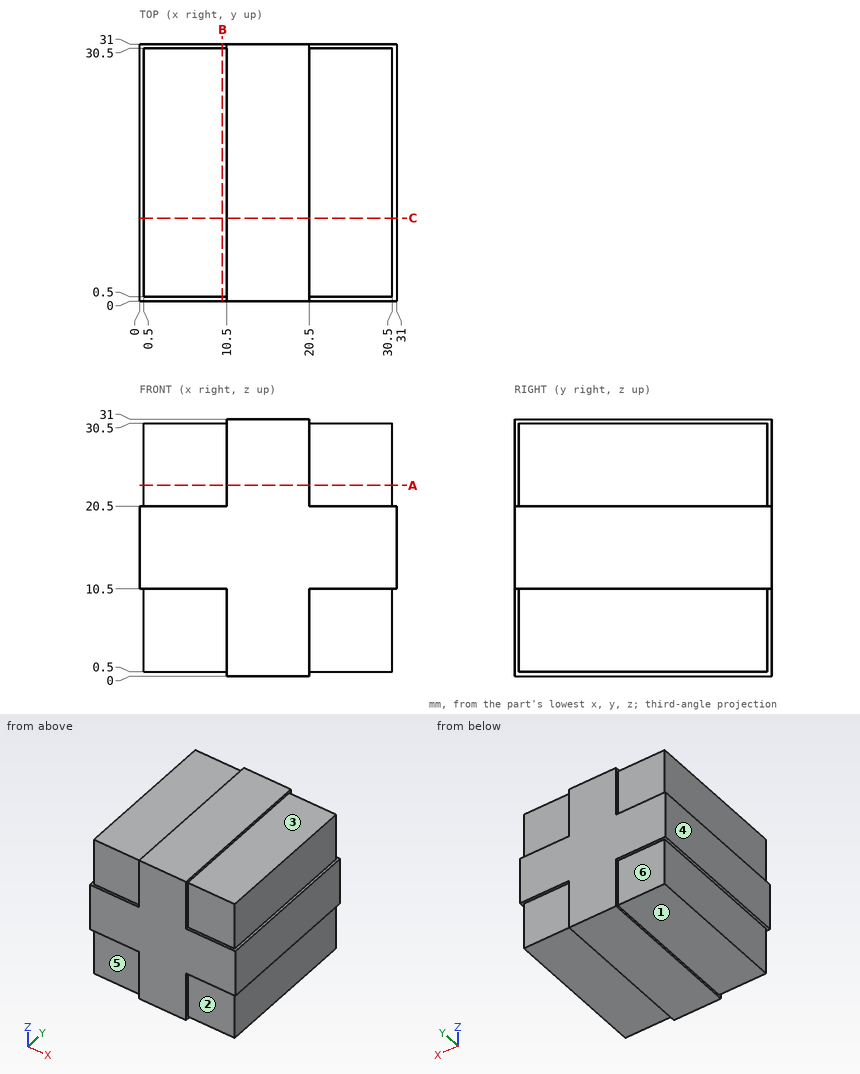
Geometry check sheet. Reference: drawing and pictorial views, mm from the part's lowest x, y, z. A direction names the side the tool comes from. Coordinates: 2 decimals unless noted, no trailing zeros. Order: outer loops, then holes, each group sorted by start corner. A loop starts at its lowest first (then second) coordinate and runs counter-clockwise, first axis right, second up. Notation, with made-up numbers: (11.25, 30) -> (55.25, 30) arc R18 ccw to (55.25, 37) -> close; hole circle Ø10 at (21.25, 79.5). An arc over 180 degrees is marked (long way). Put each result on its own line as item: value. Start each with the question number.
1) Cross-section at C-C (y = 10). Enter the section's corners in (x, z), plus the area to 3 significant figures.
2) Cross-section at B-B (x = 10). Enter the section's corners in (y, z), plus the area to 3 significant figures.
3) Cross-section at A-A (z = 23). Enter the section's corners in (x, y).
4) Release check for a two-part mould opening along Y. For the marked faces 4, 5 and 6 record: pulls with the +Y half, pulls with the -Y half, needs draft (parallel to the pull), parting line crosses it, or undercut.
5) Material ranges on L1, parallel to Y at x = 30, z = 8.5, recorded low to high.
6) Tool access check on the marked faces 1, 2 and 3. Record the directions out of +Z, -Z, +X, -X, +Y, -Y that give a thin tool (end or side, any length) a straight path to the whole face; none if there is none.
7) Go/stop test with flat-tipped pins: pin 1 (3 mm diameter, centred on x = 6.5, z = 6.5, fed in from +Y); pin 2 (12 mm diameter, centred on x = 15.5, z = 22, fed in from -Y); pin 3 (11 mm diameter, centred on x = 27, z = 3.5, fed in from -Y); pin 4 (3 mm diameter, centred on y = 8.5, z = 7.5, fed in from -X). Record where each tip stops, or that it passes through.
Geometry check:
1. outline: (0, 10.5) -> (0.5, 10.5) -> (0.5, 0.5) -> (10.5, 0.5) -> (10.5, 0) -> (20.5, 0) -> (20.5, 0.5) -> (30.5, 0.5) -> (30.5, 10.5) -> (31, 10.5) -> (31, 20.5) -> (30.5, 20.5) -> (30.5, 30.5) -> (20.5, 30.5) -> (20.5, 31) -> (10.5, 31) -> (10.5, 30.5) -> (0.5, 30.5) -> (0.5, 20.5) -> (0, 20.5) -> close
1. area: 920 mm^2
2. outline: (0, 10.5) -> (0.5, 10.5) -> (0.5, 0.5) -> (30.5, 0.5) -> (30.5, 10.5) -> (31, 10.5) -> (31, 20.5) -> (30.5, 20.5) -> (30.5, 30.5) -> (0.5, 30.5) -> (0.5, 20.5) -> (0, 20.5) -> close
2. area: 910 mm^2
3. outline: (0.5, 0.5) -> (10.5, 0.5) -> (10.5, 0) -> (20.5, 0) -> (20.5, 0.5) -> (30.5, 0.5) -> (30.5, 30.5) -> (20.5, 30.5) -> (20.5, 31) -> (10.5, 31) -> (10.5, 30.5) -> (0.5, 30.5) -> close
4. face 4: needs draft
4. face 5: pulls with the -Y half
4. face 6: pulls with the +Y half
5. L1: y = 0.5 to 30.5
6. face 1: -Z, -X, +Y, -Y
6. face 2: -Z, +X, -Y
6. face 3: +Z, +X, +Y, -Y
7. pin 1: stops at y = 30.5
7. pin 2: stops at y = 0
7. pin 3: stops at y = 0.5
7. pin 4: stops at x = 0.5
